Work out the finished part from the listing and answer in its coordinate system (mm). A direction names the side the tool comes from. Give positions to 0.01 mm unless a question says otherwise; leave off trailing zeros. Order: outer loops, then holes, each group sorted by start corner. A loop starts at its lowest first (then second) coordinate and runs counter-clockwise, first axis right, second up. Notation, with made-up numbers: (11.5, -24.5) - (66.5, -24.5) arc R14 ccw to (66.5, 0.5) - close; hole circle Ø4 at (61, -4). An arc over 180 degrees is marked (long way). Put each result on its own line as item: value.
```python
from build123d import *

# Parameters (mm, degrees)
F0_W      = 50.8
F0_H      = 50.8
F1_DEPTH  = 101.6
F3_DEPTH  = 12.7
F5_DEPTH  = 25.4
F7_DEPTH  = 8.89
F8_W      = 50.8
F8_H      = 50.8
F9_DEPTH  = 2.286
F10_R     = 19.05
F11_DEPTH = 16.51
F11_TAPER = 20
F12_R     = 9.525
F13_DEPTH = 25.4
F14_R     = 5.08
F15_R     = 5.08


with BuildPart() as f1:
    # F0 (on Front) → F1 (new body)
    with BuildSketch(Plane.XZ):
        with Locations((-25.4, 25.4)):
            Rectangle(F0_W, F0_H)
        Polygon((-48.26, 12.192), (-48.26, 48.26), (-2.54, 48.26), (-2.54, 12.1909337732), (-9.652, 12.1909337732), (-9.652, 9.6509337732), (-7.112, 9.6509337732), (-7.112, 7.1109337732), (-9.6097155579, 7.1109337732), (-9.6097155579, 2.54), (-41.1057155579, 2.54), (-41.1057155579, 7.112), (-43.688, 7.112), (-43.688, 9.652), (-41.148, 9.652), (-41.148, 12.192), align=None, mode=Mode.SUBTRACT)
    extrude(amount=F1_DEPTH)

    # F2 (on face) → F3 (cut)
    with BuildSketch(Plane(origin=(-50.8, 0, 0), x_dir=(0, -1, 0), z_dir=(-1, 0, 0))):
        with BuildLine():
            ThreePointArc((63.5, 25.4), (57.15, 31.75), (50.8, 25.4))
            Line((50.8, 25.4), (63.5, 25.4))
        make_face()
        with BuildLine():
            ThreePointArc((88.9, 25.4), (82.55, 31.75), (76.2, 25.4))
            Line((76.2, 25.4), (88.9, 25.4))
        make_face()
        with BuildLine():
            Line((88.9, 25.4), (76.2, 25.4))
            ThreePointArc((76.2, 25.4), (82.55, 19.05), (88.9, 25.4))
        make_face()
        with BuildLine():
            Line((63.5, 25.4), (50.8, 25.4))
            ThreePointArc((50.8, 25.4), (57.15, 19.05), (63.5, 25.4))
        make_face()
    extrude(amount=-F3_DEPTH, mode=Mode.SUBTRACT)

    # F4 (on face) → F5 (cut)
    with BuildSketch(Plane(origin=(0, 0, 0), x_dir=(1, 0, 0), z_dir=(0, 0, -1))):
        with BuildLine():
            ThreePointArc((-25.4, 29.21), (-35.56, 19.05), (-25.4, 8.89))
            Line((-25.4, 8.89), (-25.4, 29.21))
        make_face()
        with BuildLine():
            ThreePointArc((-25.4, 92.71), (-35.56, 82.55), (-25.4, 72.39))
            Line((-25.4, 72.39), (-25.4, 92.71))
        make_face()
        with BuildLine():
            Line((-25.4, 92.71), (-25.4, 72.39))
            ThreePointArc((-25.4, 72.39), (-18.2157951031, 75.3657951031), (-15.24, 82.55))
            ThreePointArc((-15.24, 82.55), (-18.2157951031, 89.7342048969), (-25.4, 92.71))
        make_face()
        with BuildLine():
            ThreePointArc((-25.4, 60.96), (-35.56, 50.8), (-25.4, 40.64))
            Line((-25.4, 40.64), (-25.4, 60.96))
        make_face()
        with BuildLine():
            Line((-25.4, 60.96), (-25.4, 40.64))
            ThreePointArc((-25.4, 40.64), (-18.2157951031, 43.6157951031), (-15.24, 50.8))
            ThreePointArc((-15.24, 50.8), (-18.2157951031, 57.9842048969), (-25.4, 60.96))
        make_face()
        with BuildLine():
            Line((-25.4, 29.21), (-25.4, 8.89))
            ThreePointArc((-25.4, 8.89), (-18.2157951031, 11.8657951031), (-15.24, 19.05))
            ThreePointArc((-15.24, 19.05), (-18.2157951031, 26.2342048969), (-25.4, 29.21))
        make_face()
    extrude(amount=-F5_DEPTH, mode=Mode.SUBTRACT)

    # F6 (on face) → F7 (join)
    with BuildSketch(Plane(origin=(0, 0, 0), x_dir=(1, 0, 0), z_dir=(0, 0, -1))):
        with BuildLine():
            ThreePointArc((-12.9565921067, 16.51), (-25.4, 6.35), (-37.8434078933, 16.51))
            Line((-37.8434078933, 16.51), (-39.1371503595, 16.51))
            ThreePointArc((-39.1371503595, 16.51), (-25.4, 5.08), (-11.6628496405, 16.51))
            Line((-11.6628496405, 16.51), (-12.9565921067, 16.51))
        make_face()
        with BuildLine():
            ThreePointArc((-12.9565921067, 48.26), (-25.4, 38.1), (-37.8434078933, 48.26))
            Line((-37.8434078933, 48.26), (-39.1371503595, 48.26))
            ThreePointArc((-39.1371503595, 48.26), (-25.4, 36.83), (-11.6628496405, 48.26))
            Line((-11.6628496405, 48.26), (-12.9565921067, 48.26))
        make_face()
        with BuildLine():
            ThreePointArc((-12.9565921067, 80.01), (-25.4, 69.85), (-37.8434078933, 80.01))
            Line((-37.8434078933, 80.01), (-39.1371503595, 80.01))
            ThreePointArc((-39.1371503595, 80.01), (-25.4, 68.58), (-11.6628496405, 80.01))
            Line((-11.6628496405, 80.01), (-12.9565921067, 80.01))
        make_face()
    extrude(amount=F7_DEPTH)

    # F8 (on face) → F9 (join)
    with BuildSketch(Plane.XZ.offset(101.6)):
        with Locations((-25.4, 25.4)):
            Rectangle(F8_W, F8_H)
    extrude(amount=F9_DEPTH)

    # F10 (on face) → F11 (join)
    with BuildSketch(Plane.XZ.offset(103.886)):
        with Locations((-25.4, 25.4)):
            Circle(F10_R)
    extrude(amount=F11_DEPTH, taper=F11_TAPER)

    # F12 (on face) → F13 (cut)
    with BuildSketch(Plane.XZ.offset(120.396)):
        with Locations((-25.4, 25.4)):
            Circle(F12_R)
    extrude(amount=-F13_DEPTH, mode=Mode.SUBTRACT)

    # F14
    f14_edges = [f1.edges().sort_by_distance(p)[0] for p in [
        (0, -51.943, 0),
        (-50.8, -51.943, 0),
        (-50.8, -51.943, 50.8),
        (0, -51.943, 50.8),
    ]]
    fillet(f14_edges, radius=F14_R)

    # F15
    f15_edges = [f1.edges().sort_by_distance(p)[0] for p in [
        (-25.4, -103.886, 50.8),
    ]]
    fillet(f15_edges, radius=F15_R)


solid = f1.part
```
(1) Given pin 1 (8 mm diameter, centred on x = -30, y = -100.5, fed in from -Z); pin 2 (10 mm diameter, centred on x = -40.5, z = 38.5, fed in from +Y); pin 3 (1 mm diameter, centred on x = -23.5, y = -102, fed in from +Z), each flat-ended and moving along its own axis, determine where each tip first touches the part or whether it passes through.
Geometry check:
pin 1: stops at z = 0
pin 2: stops at y = -101.6
pin 3: stops at z = 50.03
(2) Section C-C, the plane z = 20.5 is taken. Count the separate pieces of the cut face and the enclosed holes in it, then the cut area to 3 significant figures.
Geometry check:
separate pieces: 4
enclosed holes: 0
area: 777 mm²
(3) A tool of negligible diameter and unlimited length cuts with its end or side. For faces 4 (the face through (-15, -50, 2.54)), 5 (the face through (-25.157, -69.852, -4.383)), 6 (the face through (-25.671, -36.833, -4.383)), from which of +Z, -Z, +X, -X, +Y, -Y can it reach the whole face along a straight path? Write none if from no direction.
Geometry check:
face 4: +Y
face 5: -Z, -Y
face 6: -Z
(4) Section A-A, the plane y = -96 is taken. Write down the section's boundary in (x, z), then the cut area to 3 significant figures.
Geometry check:
outline: (-50.8, 5.08) arc R5.08 ccw to (-45.72, 0) - (-5.08, 0) arc R5.08 ccw to (0, 5.08) - (0, 45.72) arc R5.08 ccw to (-5.08, 50.8) - (-45.72, 50.8) arc R5.08 ccw to (-50.8, 45.72) - close; hole (-48.26, 12.19) - (-41.15, 12.19) - (-41.15, 9.65) - (-43.69, 9.65) - (-43.69, 7.11) - (-41.11, 7.11) - (-41.11, 2.54) - (-9.61, 2.54) - (-9.61, 7.11) - (-7.11, 7.11) - (-7.11, 9.65) - (-9.65, 9.65) - (-9.65, 12.19) - (-2.54, 12.19) - (-2.54, 48.26) - (-48.26, 48.26) - close
area: 593 mm²
(5) Straight lines are drawn through the part: line 1 (Z direction, x = -9, y = -72); line 2 (X direction, y = -18, z = 27); line 3 (Z direction, x = -16.5, y = -35.5). For each, find the intervals that lie inside material, in ascending order.
Geometry check:
line 1: z = 0 to 7.11, 9.65 to 12.19, 48.26 to 50.8
line 2: x = -50.8 to -48.26, -2.54 to 0
line 3: z = 0 to 2.54, 48.26 to 50.8
(6) Determine the mould class of faces 1 (the face through (-1.53, -102.44, 25.12)), 2 (the face through (-6, -50, 12.191)), 3 (the face through (-1.528, -50.095, 1.449)) for opening direction Z: pulls with the +Z half, pulls with the -Z half, needs draft (parallel to the pull), parting line crosses it, or undercut.
Geometry check:
face 1: needs draft
face 2: undercut
face 3: pulls with the -Z half
